Here's how the part is built. I have some questions about the finished solid (model axes, mm). Face numbers are marked on the shaded views. Round coordinates to 2 decimals unless told otherwise and drop trailing zeros. Order: outer loops, then holes, each group sorted by start corner. A loop starts at its lowest first (then second) coordinate and runs counter-clockwise, first axis right, second up. Notation, with made-up numbers: (83.5, 61.5) - (132.5, 61.5) arc R6 ccw to (132.5, 67.5) - close; hole circle Ø5 at (73.25, -26). An arc over 180 degrees is marked (long way). One line per item, written item: value.
from build123d import *

# Parameters (mm, degrees)
SKETCH1_W                       = 63.5
SKETCH1_H                       = 63.5
BOSS_EXTRUDE1_DEPTH             = 9.525
SKETCH2_R                       = 20.6375
CUT_EXTRUDE1_DEPTH              = 46.900442536
F_10_32_TAPPED_HOLE1_AT_2_COUNT = 2
F_10_32_TAPPED_HOLE1_AT_2_PITCH = 16.9164
F_10_32_TAPPED_HOLE1_AT_3_COUNT = 2
F_10_32_TAPPED_HOLE1_AT_3_PITCH = 33.6804
F_10_32_TAPPED_HOLE1_AT_4_COUNT = 2
F_10_32_TAPPED_HOLE1_AT_4_PITCH = 16.764
F_10_0_1935_DIAMETER_HOLE1_D    = 5.334


with BuildPart() as part:
    # Sketch1 → Boss-Extrude1 (new body)
    with BuildSketch(Plane(origin=(0, 0, 0), x_dir=(-1, 0, 0), z_dir=(0, 0, -1))):
        Rectangle(SKETCH1_W, SKETCH1_H)
    extrude(amount=-BOSS_EXTRUDE1_DEPTH)

    # Sketch2 → Cut-Extrude1 (cut, through all)
    with BuildSketch(Plane.XY.offset(9.525)):
        Circle(SKETCH2_R)
    extrude(amount=-CUT_EXTRUDE1_DEPTH, mode=Mode.SUBTRACT)

    # Sketch3 → #10-32 Tapped Hole1 (revolve, cut)
    with BuildSketch(Plane(origin=(8.4582, -31.75, 4.7625), x_dir=(0, 0, -1), z_dir=(1, 0, 0))):
        Polygon((0, 0), (0, 13.913317848), (2.0193, 12.7), (2.0193, 0), align=None)
    f_10_32_tapped_hole1 = revolve(axis=Axis((8.4582, -38.1, 4.7625), (0, 1, 0)), mode=Mode.SUBTRACT)

    # #10-32 Tapped Hole1 at 2: #10-32 Tapped Hole1 ×2
    with Locations(*[(-i * F_10_32_TAPPED_HOLE1_AT_2_PITCH, 0, 0) for i in range(1, F_10_32_TAPPED_HOLE1_AT_2_COUNT)]):
        add(f_10_32_tapped_hole1, mode=Mode.SUBTRACT)

    # #10-32 Tapped Hole1 at 3: #10-32 Tapped Hole1 ×2
    with Locations(*[(-i * F_10_32_TAPPED_HOLE1_AT_3_PITCH, 0, 0) for i in range(1, F_10_32_TAPPED_HOLE1_AT_3_COUNT)]):
        add(f_10_32_tapped_hole1, mode=Mode.SUBTRACT)

    # #10-32 Tapped Hole1 at 4: #10-32 Tapped Hole1 ×2
    with Locations(*[(i * F_10_32_TAPPED_HOLE1_AT_4_PITCH, 0, 0) for i in range(1, F_10_32_TAPPED_HOLE1_AT_4_COUNT)]):
        add(f_10_32_tapped_hole1, mode=Mode.SUBTRACT)

    # #10 (0.1935) Diameter Hole1 (through all)
    with Locations(Plane(origin=(0, 0, 0), x_dir=(-1, 0, 0), z_dir=(0, 0, -1))):
        with Locations((-20.622229928, 11.90625), (-20.622229928, -11.90625), (0, -23.8125), (20.622229928, -11.90625), (20.622229928, 11.90625), (0, 23.8125)):
            Hole(F_10_0_1935_DIAMETER_HOLE1_D / 2)

    # Mirror1: #10-32 Tapped Hole1 across plane
    add(f_10_32_tapped_hole1.mirror(Plane.ZX), mode=Mode.SUBTRACT)

    # Mirror1 copy 1 sketch → Mirror1 copy 1 (revolve, cut)
    with BuildSketch(Plane(origin=(-8.4582, 31.75, 4.7625), x_dir=(0, 0, -1), z_dir=(1, 0, 0))):
        Polygon((0, 0), (0, -13.913317848), (2.0193, -12.7), (2.0193, 0), align=None)
    revolve(axis=Axis((-8.4582, 38.1, 4.7625), (0, 1, 0)), mode=Mode.SUBTRACT)

    # Mirror1 copy 2 sketch → Mirror1 copy 2 (revolve, cut)
    with BuildSketch(Plane(origin=(-25.2222, 31.75, 4.7625), x_dir=(0, 0, -1), z_dir=(1, 0, 0))):
        Polygon((0, 0), (0, -13.913317848), (2.0193, -12.7), (2.0193, 0), align=None)
    revolve(axis=Axis((-25.2222, 38.1, 4.7625), (0, 1, 0)), mode=Mode.SUBTRACT)

    # Mirror1 copy 3 sketch → Mirror1 copy 3 (revolve, cut)
    with BuildSketch(Plane(origin=(25.2222, 31.75, 4.7625), x_dir=(0, 0, -1), z_dir=(1, 0, 0))):
        Polygon((0, 0), (0, -13.913317848), (2.0193, -12.7), (2.0193, 0), align=None)
    revolve(axis=Axis((25.2222, 38.1, 4.7625), (0, 1, 0)), mode=Mode.SUBTRACT)


solid = part.part
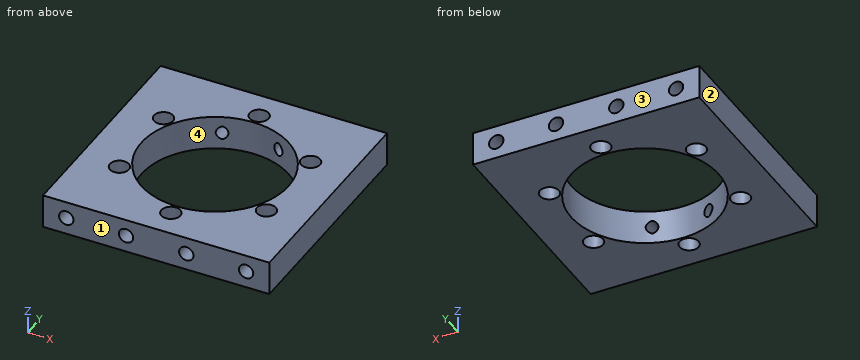
Q1. If we section it at A-A, the plane x = 0: Give the number of separate pieces and of enclosed holes in the cut face, then the cut area to 3 significant figures.
Results list:
separate pieces: 4
enclosed holes: 0
area: 110 mm²
Q2. If I drill on line 1 along Y through (x, z) = (0, 6.75); line 2 along X through (y, z) = (25, 5.75); line 3 along X through (y, z) = (21, 3.5), over which ranges is the centre line in solid material (lowest first)?
Results list:
line 1: -31.75 to -26.48, -21.15 to -20.64, 20.64 to 21.15, 26.48 to 31.75
line 2: -31.75 to -26.98, -23.46 to -10.22, -6.7 to -2.39, 2.39 to 6.7, 10.22 to 23.46, 26.98 to 31.75
line 3: -31.75 to -26.8, -23.65 to -10.03, -6.88 to 6.88, 10.03 to 23.65, 26.8 to 31.75
Q3. If we section it at C-C, the plane y = 10: Please give me the cut outline in (x, z) (3 decimals).
Results list:
outline: (-31.75, 0) - (-22.487, 0) - (-22.487, 9.525) - (-31.75, 9.525) - close; (-18.757, 0) - (-18.053, 0) - (-18.053, 9.525) - (-18.757, 9.525) - close; (18.053, 0) - (18.757, 0) - (18.757, 9.525) - (18.053, 9.525) - close; (22.487, 0) - (31.75, 0) - (31.75, 9.525) - (22.487, 9.525) - close
Q4. We'd pull the mould along Y, two halves only. Please class the marked faces 1, 2, 3 and 4: released by +Y, released by -Y, zero draft, split by the parting line, or undercut.
Results list:
face 1: released by -Y
face 2: zero draft
face 3: released by +Y
face 4: undercut
Q5. Will these pins go through, and if not, where does the flat tip stop? pin 1 (3 mm diameter, centred on x = 25.22, z = 4.76, fed in from +Y); pin 2 (5.5 mm diameter, centred on x = 8.46, z = 4.76, fed in from +Y); pin 3 (2.5 mm diameter, centred on x = -25.22, z = 4.76, fed in from +Y); pin 4 (3.5 mm diameter, centred on x = 25.22, z = 4.76, fed in from +Y).
Results list:
pin 1: y = 18.74
pin 2: y = 31.75
pin 3: y = 18.59
pin 4: y = 18.89
